from build123d import *

# Parameters (mm, degrees)
SKETCH1_R           = 35
SKETCH1_R_2         = 5
SKETCH1_R_3         = 2.5
BOSS_EXTRUDE1_DEPTH = 10
SKETCH2_R           = 16
CUT_EXTRUDE1_DEPTH  = 5
SKETCH5_R           = 13
CUT_EXTRUDE2_DEPTH  = 5
BOSS_EXTRUDE2_START = 35
SKETCH6_R           = 17.5
SKETCH6_R_2         = 13
BOSS_EXTRUDE2_DEPTH = 35


with BuildPart() as part:
    # Sketch1 → Boss-Extrude1 (new body)
    with BuildSketch(Plane(origin=(0, 0, 0), x_dir=(1, 0, 0), z_dir=(0, 1, 0))):
        with Locations(Location((0, 0, 0), (0, 0, 270))):
            Circle(SKETCH1_R)
        with Locations(Location((0, 0, 0), (0, 0, 270))):
            Circle(SKETCH1_R_2, mode=Mode.SUBTRACT)
        with Locations(Location((0, 22.5, 0), (0, 0, 270))):
            Circle(SKETCH1_R_3, mode=Mode.SUBTRACT)
        with Locations(Location((19.485571585, 11.25, 0), (0, 0, 270))):
            Circle(SKETCH1_R_3, mode=Mode.SUBTRACT)
        with Locations(Location((19.485571585, -11.25, 0), (0, 0, 270))):
            Circle(SKETCH1_R_3, mode=Mode.SUBTRACT)
        with Locations(Location((0, -22.5, 0), (0, 0, 270))):
            Circle(SKETCH1_R_3, mode=Mode.SUBTRACT)
        with Locations(Location((-19.485571585, -11.25, 0), (0, 0, 270))):
            Circle(SKETCH1_R_3, mode=Mode.SUBTRACT)
        with Locations(Location((-19.485571585, 11.25, 0), (0, 0, 270))):
            Circle(SKETCH1_R_3, mode=Mode.SUBTRACT)
    extrude(amount=BOSS_EXTRUDE1_DEPTH)

    # Sketch2 → Cut-Extrude1 (cut)
    with BuildSketch(Plane.XZ):
        with Locations(Location((0, 0, 0), (0, 0, 270))):
            Circle(SKETCH2_R)
    extrude(amount=-CUT_EXTRUDE1_DEPTH, mode=Mode.SUBTRACT)

    # Sketch5 → Cut-Extrude2 (cut)
    with BuildSketch(Plane(origin=(0, 10, 0), x_dir=(1, 0, 0), z_dir=(0, 1, 0))):
        with Locations(Location((0, 0, 0), (0, 0, 270))):
            Circle(SKETCH5_R)
    extrude(amount=-CUT_EXTRUDE2_DEPTH, mode=Mode.SUBTRACT)

    # Sketch6 → Boss-Extrude2 (add)
    with BuildSketch(Plane(origin=(0, 10, 0), x_dir=(1, 0, 0), z_dir=(0, 1, 0)).offset(BOSS_EXTRUDE2_START)):
        with Locations(Location((0, 0, 0), (0, 0, 270))):
            Circle(SKETCH6_R)
        with Locations(Location((0, 0, 0), (0, 0, 270))):
            Circle(SKETCH6_R_2, mode=Mode.SUBTRACT)
    extrude(amount=-BOSS_EXTRUDE2_DEPTH)


solid = part.part
Build history of the part. All positions in model axes, mm. A direction names the side the tool comes from. Give positions to 0.01 mm unless a question says otherwise; leave off trailing zeros. Order: outer loops, then holes, each group sorted by start corner. A loop starts at its lowest first (then second) coordinate and runs counter-clockwise, first axis right, second up. Notation, with made-up numbers: M -19,39 L 5,39 A33 ccw 5,69 Z; hole C -23.75,48 d8. An arc over 180 degrees is marked long. Use one line per item in the form item = value.
Q1. Slice it at D-D, the plane z = -11. Write the cut outline in (x, y), and give its area (3 significant figures).
Conclusion:
outline = M -33.23,0 L -21.97,0 L -21.97,10 L -33.23,10 Z; M -17,0 L -11.62,0 L -11.62,5 L -6.93,5 L -6.93,45 L -13.61,45 L -13.61,10 L -17,10 Z; M 6.93,5 L 11.62,5 L 11.62,0 L 17,0 L 17,10 L 13.61,10 L 13.61,45 L 6.93,45 Z; M 21.97,0 L 33.23,0 L 33.23,10 L 21.97,10 Z
area = 847 mm2
Q2. Which spindle directions (+Z, -Z, +X, -X, +Y, -Y) get a long thin tool onto all of the face, cutting with end or side? Do faces 1 (the flat face through (13.1, 5, 1.3)), 2 (the cylindrical face through (-10.648, 27.745, -13.887)), 3 (the cylindrical face through (-7.91, 25.28, -10.316)). Say none if no direction does.
Conclusion:
face_1 = -Y
face_2 = +Y
face_3 = +Y, -Y
Q3. Pin check, flat tips, straight feed: P1, Ø16, axis at x = 0, z = 5.5, coming from the -Y side; P2, Ø3, axis at x = -27.5, z = -7.5, coming from the +Y side; P3, Ø4, axis at y = 20, z = -7, coming from the +X side; P4, Ø6, axis at x = -19.49, z = 11.25, coming from the -Y side. Stop position of each tip, or through.
Conclusion:
P1 = 5
P2 = 10
P3 = 16.77
P4 = 0
Q4. Slice it at C-C, the plane x = 20.5. Write the cut outline in (y, z).
Conclusion:
outline = M 0,-28.37 L 10,-28.37 L 10,-13.53 L 0,-13.53 Z; M 0,-8.97 L 10,-8.97 L 10,8.97 L 0,8.97 Z; M 0,13.53 L 10,13.53 L 10,28.37 L 0,28.37 Z
Q5. Pull direction Z, two halves, no side cores. Call faces 4 (the flat face through (8, 10, -16)), 5 (the cylindrical face through (-21, 5, -28)), 6 (the cylindrical face through (0, 5, -25)): released by +Z, released by -Z, zero draft, split by the parting line, or undercut.
Conclusion:
face_4 = zero draft
face_5 = split by the parting line
face_6 = undercut
Q6. Wall check: probe 1 along X at (y, z) = (3.2, 0); probe 2 along X at (y, z) = (6.5, -11.25); probe 3 along X at (y, z) = (4, -11). Give the ranges that are in metal, low to high.
Conclusion:
probe_1 = -35 to -16, 16 to 35
probe_2 = -33.14 to -21.99, -16.99 to -6.51, 6.51 to 16.99, 21.99 to 33.14
probe_3 = -33.23 to -21.97, -17 to -11.62, 11.62 to 17, 21.97 to 33.23
Q7. Slice it at A-A, the plane z = 0. Write the cut outline in (x, y), and give its area (3 significant figures).
Conclusion:
outline = M -35,0 L -16,0 L -16,5 L -13,5 L -13,45 L -17.5,45 L -17.5,10 L -35,10 Z; M 13,5 L 16,5 L 16,0 L 35,0 L 35,10 L 17.5,10 L 17.5,45 L 13,45 Z
area = 725 mm2
Q8. Slice it at B-B, the plane x = 0. Write the cut outline in (y, z).
Conclusion:
outline = M 0,-35 L 10,-35 L 10,-25 L 0,-25 Z; M 0,-20 L 10,-20 L 10,-17.5 L 45,-17.5 L 45,-13 L 5,-13 L 5,-16 L 0,-16 Z; M 0,16 L 5,16 L 5,13 L 45,13 L 45,17.5 L 10,17.5 L 10,20 L 0,20 Z; M 0,25 L 10,25 L 10,35 L 0,35 Z
